```python
from build123d import *

# Parameters (mm, degrees)
SKETCH1_R           = 8
BOSS_EXTRUDE1_DEPTH = 2
SKETCH2_R           = 6
BOSS_EXTRUDE2_DEPTH = 5
SKETCH3_R           = 2
CUT_EXTRUDE1_DEPTH  = 2
SKETCH4_R           = 0.35
CUT_EXTRUDE2_DEPTH  = 14.304134696
CHAMFER2_SIZE       = 2


with BuildPart() as part:
    # Sketch1 → Boss-Extrude1 (new body)
    with BuildSketch(Plane.XY):
        Circle(SKETCH1_R)
    extrude(amount=BOSS_EXTRUDE1_DEPTH)

    # Sketch2 → Boss-Extrude2 (add)
    with BuildSketch(Plane.XY.offset(2)):
        Circle(SKETCH2_R)
    extrude(amount=BOSS_EXTRUDE2_DEPTH)

    # Sketch3 → Cut-Extrude1 (cut)
    with BuildSketch(Plane(origin=(0, 0, 0), x_dir=(-1, 0, 0), z_dir=(0, 0, -1))):
        Circle(SKETCH3_R)
    extrude(amount=-CUT_EXTRUDE1_DEPTH, mode=Mode.SUBTRACT)

    # Sketch4 → Cut-Extrude2 (cut, through all)
    with BuildSketch(Plane.XY.offset(7)):
        Circle(SKETCH4_R)
    extrude(amount=-CUT_EXTRUDE2_DEPTH, mode=Mode.SUBTRACT)

    # Chamfer2
    # the kernel refuses this chamfer: 2 mm, written as the material it takes off along each edge
    with BuildSketch(Plane(origin=(0, 0, 2), x_dir=(1, 0, 0), z_dir=(0, -1, 0))) as chamfer2_piece_1_section:
        Polygon((0.35 + CHAMFER2_SIZE, 0), (0.35, CHAMFER2_SIZE), (0.35, 0), align=None)
    chamfer2_piece_1 = revolve(axis=Axis((0, 0, 2), (0, 0, 1)), mode=Mode.PRIVATE)
    chamfer2_piece_1 = chamfer2_piece_1 & Plane(origin=(0, 0, 3.186782056), x_dir=(-1, 0, 0), z_dir=(0, 0, -1)) * Cylinder(2, 10, mode=Mode.PRIVATE)
    add(chamfer2_piece_1, mode=Mode.SUBTRACT)


solid = part.part
```
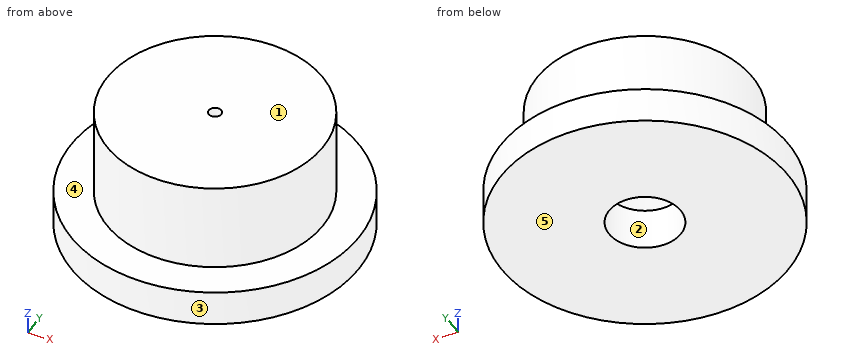
The model under review builds one solid part; all positions refer to its coordinate system, in mm. Face numbers are marked on the shaded views. A direction names the side the tool comes from. Round coordinates to 2 decimals unless told otherwise and drop trailing zeros. Loops run counter-clockwise (first coordinate to the right, second up) from the corner with the lowest first, then second, coordinate; pieces in that order, holes last. Notation, with made-up numbers: (73.25, -25.5) -> (123.25, -25.5) arc R17 ccw to (123.25, -1.5) -> close; hole circle Ø3 at (80, -26.75). An arc over 180 degrees is marked (long way). Answer as a JSON object with one key per item and string values. Group by question number.
1) For pin 1 Ø1 at (x, z) = (0, 5.5) entering from -Y; pin 2 Ø1.5 at (y, z) = (1, 4) entering from -X, all flat-tipped, find the tip position at first contact; note any pin that passes through.
2) We need section D-D on x = 3.25. Write out the cut boundary in (y, z), then the cut area to 3 significant figures.
3) We need section A-A on x = 0. Write out the cut boundary in (y, z).
4) We need section C-C on z = 3.75. Write out the cut boundary in (x, y), then the cut area to 3 significant figures.
5) Mouldability with a two-part tool opening along X and no side actions: class the marked faces 1, 2 and 3 as released by +X, released by -X, zero draft, split by the parting line, or undercut.
6) For the marked faces 4 and 5, list the 3-axis set-ups (+Z, -Z, +X, -X, +Y, -Y) from which the entire face can be reached by the end or side of a thin tool; tool diameter is ignored.
7) For line 1 (Y direction, x = 0, z = 1.25); line 2 (Z direction, x = -6.75, y = -2.5); line 3 (Y direction, x = -4.75, z = 0.5), list the stretches that pass through material, from the lowest coordinate up. Write a range as [from, to].
Result set:
{
 "1": {"pin 1": "y = -6", "pin 2": "x = -5.99"},
 "2": {"outline": "(-7.31, 0) -> (7.31, 0) -> (7.31, 2) -> (5.04, 2) -> (5.04, 7) -> (-5.04, 7) -> (-5.04, 2) -> (-7.31, 2) -> close", "area": "79.7 mm²"},
 "3": {"outline": "(-8, 0) -> (-2, 0) -> (-2, 2.35) -> (-0.35, 4) -> (-0.35, 7) -> (-6, 7) -> (-6, 2) -> (-8, 2) -> close; (0.35, 4) -> (2, 2.35) -> (2, 0) -> (8, 0) -> (8, 2) -> (6, 2) -> (6, 7) -> (0.35, 7) -> close"},
 "4": {"outline": "circle Ø12 at (0, 0); hole circle Ø1.2 at (0, 0)", "area": "112 mm²"},
 "5": {"face 1": "zero draft", "face 2": "undercut", "face 3": "split by the parting line"},
 "6": {"face 4": "+Z", "face 5": "-Z, +X, -X, +Y, -Y"},
 "7": {"line 1": "[-8, -2], [2, 8]", "line 2": "[0, 2]", "line 3": "[-6.44, 6.44]"}
}
